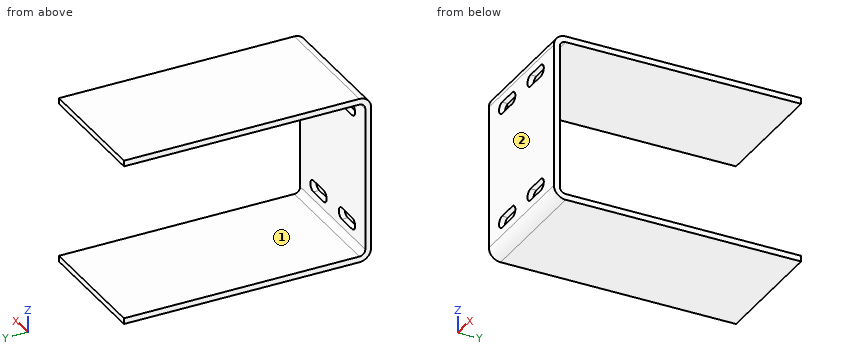
```python
from build123d import *

# Parameters (mm, degrees)
F1_DEPTH = 64
F3_DEPTH = 3


with BuildPart() as f1:
    # F0 (on Right) → F1 (new body)
    with BuildSketch(Plane.YZ):
        with BuildLine():
            Line((0, 80), (0, 6))
            ThreePointArc((0, 6), (1.757359, 1.757359), (6, 0))
            Line((6, 0), (127, 0))
            Line((127, 0), (127, 3))
            Line((127, 3), (6, 3))
            ThreePointArc((6, 3), (3.87868, 3.87868), (3, 6))
            Line((3, 6), (3, 80))
            ThreePointArc((3, 80), (3.87868, 82.12132), (6, 83))
            Line((6, 83), (127, 83))
            Line((127, 83), (127, 86))
            Line((127, 86), (6, 86))
            ThreePointArc((6, 86), (1.757359, 84.242641), (0, 80))
        make_face()
    extrude(amount=F1_DEPTH)

    # F2 (on face) → F3 (cut, through all)
    with BuildSketch(Plane.XZ):
        with BuildLine():
            ThreePointArc((13, 76), (10, 73), (13, 70))
            Line((13, 70), (23, 70))
            ThreePointArc((23, 70), (26, 73), (23, 76))
            Line((23, 76), (13, 76))
        make_face()
        with BuildLine():
            Line((51, 76), (41, 76))
            ThreePointArc((41, 76), (38, 73), (41, 70))
            Line((41, 70), (51, 70))
            ThreePointArc((51, 70), (54, 73), (51, 76))
        make_face()
        with BuildLine():
            ThreePointArc((41, 16), (38, 13), (41, 10))
            Line((41, 10), (51, 10))
            ThreePointArc((51, 10), (54, 13), (51, 16))
            Line((51, 16), (41, 16))
        make_face()
        with BuildLine():
            Line((23, 16), (13, 16))
            ThreePointArc((13, 16), (10, 13), (13, 10))
            Line((13, 10), (23, 10))
            ThreePointArc((23, 10), (26, 13), (23, 16))
        make_face()
    extrude(amount=-F3_DEPTH, mode=Mode.SUBTRACT)


solid = f1.part
```
Could you check a few things on this model? Use its own coordinates, in mm. Face numbers are marked on the shaded views. A direction names the side the tool comes from. Round coordinates to 2 decimals unless told otherwise and drop trailing zeros. Write each loop counter-clockwise with the first axis right and the second up, starting at its lowest first coordinate (ties: lowest second). Pieces come first, ordered by that corner, then holes. Notation, with made-up numbers: M 84,85 L 117,85 A23 ccw 117,102 Z; hole C 38.5,13 d2. An arc over 180 degrees is marked long. Write each question's results on one line, items separated by ' | '. Start each with the question number.
1. Imagine slicing it at C-C on x = 28.5. List the corners of the cut face in (y, z) for me, and give its area (3 significant figures).
2. I'm going to push flat-ended pins straight in: pin 1 Ø0.9 at (x, y) = (16, 1.5) entering from -Z; pin 2 Ø0.9 at (x, y) = (18, 1.5) entering from +Z; pin 3 Ø8 at (x, z) = (10.5, 13) entering from +Y. Where does each tip first touch, or does it pass through?
3. Imagine slicing it at D-D on z = 49.5. List the corners of the cut face in (x, y) for me.
4. Imagine slicing it at A-A on z = 73. List the corners of the cut face in (x, y) for me, and give its area (3 significant figures).
5. Imagine slicing it at B-B on y = 78. List the corners of the cut face in (x, z) for me, and give its area (3 significant figures).
6. On a 3-axis mill with a long thin cutter (end or side, diameter ignored), from which of +Z, -Z, +X, -X, +Y, -Y can I reach the whole of each face in a straight line? I mean the marked faces 1 and 2. Say none if no direction works.
7. I need wall thicknesses on L1, parallel to Z at x = 19.5, y = 46; L2, parallel to Y at x = 17.5, z = 45.5. Which ranges of each line are inside material? Lowest first, please. Write a range as from..to.
Result sheet:
1) outline: M 0,6 A6 ccw 6,0 L 127,0 L 127,3 L 6,3 A3 cw 3,6 L 3,80 A3 cw 6,83 L 127,83 L 127,86 L 6,86 A6 ccw 0,80 Z | area: 990 mm^2
2) pin 1: stops at z = 1.57 | pin 2: stops at z = 84.43 | pin 3: stops at y = 3
3) outline: M 0,0 L 64,0 L 64,3 L 0,3 Z
4) outline: M 0,0 L 10,0 L 10,3 L 0,3 Z; M 26,0 L 38,0 L 38,3 L 26,3 Z; M 54,0 L 64,0 L 64,3 L 54,3 Z | area: 96.0 mm^2
5) outline: M 0,0 L 64,0 L 64,3 L 0,3 Z; M 0,83 L 64,83 L 64,86 L 0,86 Z | area: 384 mm^2
6) face 1: +X, -X, +Y | face 2: +Z, -Z, +X, -X, -Y
7) L1: z = 0..3, 83..86 | L2: y = 0..3
